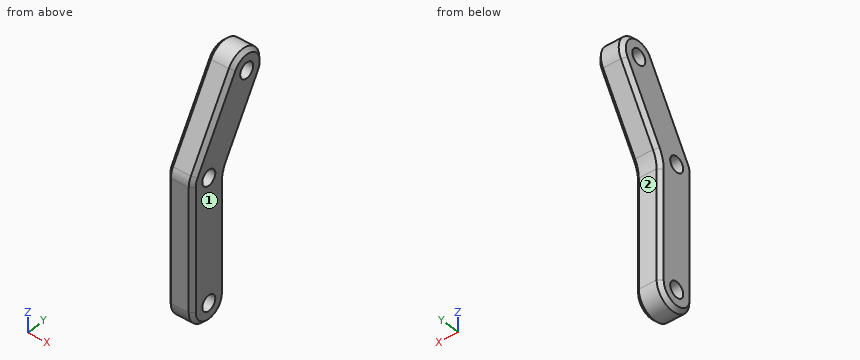
```python
from build123d import *

# Parameters (mm, degrees)
SKETCH_1_R      = 1.2
EXTRUDE_1_DEPTH = 2
FILLET_1_R      = 5
CHAMFER_1_SIZE  = 0.6


with BuildPart() as part:
    # Sketch 1 → Extrude 1 (new body, symmetric)
    with BuildSketch(Plane(origin=(0, 0, 0), x_dir=(0, 0, -1), z_dir=(1, 0, 0))):
        with BuildLine():
            Line((19, -3), (0, -3))
            ThreePointArc((0, -3), (-0.776457135, -2.897777479), (-1.5, -2.598076211))
            Line((-1.5, -2.598076211), (-13.624355653, 4.401923789))
            ThreePointArc((-13.624355653, 4.401923789), (-14.722431864, 8.5), (-10.624355653, 9.598076211))
            Line((-10.624355653, 9.598076211), (0.803847577, 3))
            Line((0.803847577, 3), (19, 3))
            ThreePointArc((19, 3), (22, 0), (19, -3))
        make_face()
        Circle(SKETCH_1_R, mode=Mode.SUBTRACT)
        with Locations((19, 0)):
            Circle(SKETCH_1_R, mode=Mode.SUBTRACT)
        with Locations((-12.124355653, 7)):
            Circle(SKETCH_1_R, mode=Mode.SUBTRACT)
    extrude(amount=EXTRUDE_1_DEPTH, both=True)

    # Fillet 1
    fillet_1_edges = [part.edges().sort_by_distance(p)[0] for p in [
        (0, 3, -0.803847577),
    ]]
    fillet(fillet_1_edges, radius=FILLET_1_R)

    # Chamfer 1
    chamfer_1_edges = [part.edges().sort_by_distance(p)[0] for p in [
        (-2, -2.897777479, 0.776457135),
        (2, 8.5, 14.722431864),
        (2, 6.633974596, 5.490381057),
        (2, 0, -22),
        (2, -3, -9.5),
        (-2, 3, -10.57179677),
        (2, 3, -10.57179677),
        (-2, 3.170370869, -0.849498314),
        (2, 3.170370869, -0.849498314),
        (2, -2.897777479, 0.776457135),
        (-2, -3, -9.5),
        (-2, 0, -22),
        (-2, 6.633974596, 5.490381057),
        (2, 0.901923789, 7.562177826),
        (-2, 8.5, 14.722431864),
        (-2, 0.901923789, 7.562177826),
    ]]
    chamfer(chamfer_1_edges, length=CHAMFER_1_SIZE)


solid = part.part
```
Work out the finished part from the listing and answer in its coordinate system (mm). Face numbers are marked on the shaded views. A direction names the side the tool comes from. Coordinates: 2 decimals unless noted, no trailing zeros. Order: outer loops, then holes, each group sorted by start corner. A loop starts at its lowest first (then second) coordinate and runs counter-clockwise, first axis right, second up. Notation, with made-up numbers: M 69,70 L 94,70 A29 ccw 94,104 Z; hole C 27.25,-4.75 d10. An arc over 180 degrees is marked long. Use CSV: the item, a comma, the result in double quotes.
1) Consider line 1 (Y direction, x = 1, z = -19); line 2 (Z direction, x = 0.3, y = 9.75); line 3 (Y direction, x = -1.15, z = -17). Determine where each line is inside the solid, lowest interval first. Write a range as [from, to].
Worked out:
line 1,"y = [-3, -1.2], [1.2, 3]"
line 2,"z = [10.93, 13.32]"
line 3,"y = [-3, 3]"
2) Section A-A on x = 1.05 is taken. Write down the section's boundary in (y, z).
Worked out:
outline,"M -3,-19 A3 ccw 3,-19 L 3,-2.14 A5 cw 3.67,0.36 L 9.6,10.62 A3 ccw 4.4,13.62 L -2.6,1.5 A3 ccw -3,0 Z; hole C 0,-19 d2.4; hole C 0,0 d2.4; hole C 7,12.12 d2.4"
3) Section C-C on y = 7 is taken. Write down the section's boundary in (x, z), plus the area to 3 significant figures.
Worked out:
outline,"M -2,7.32 L -1.4,6.12 L 1.4,6.12 L 2,7.32 L 2,10.92 L -2,10.92 Z; M -2,13.32 L 2,13.32 L 2,14.52 L 1.4,15.12 L -1.4,15.12 L -2,14.52 Z"
area,"25.3 mm^2"
4) For the marked faces 1 and 2, determine the directions among +Z, -Z, +X, -X, +Y, -Y from which every point of the face is accessible in a straight line to the end or side of a thin tool.
Worked out:
face 1,"+Z, -Z, +X, +Y, -Y"
face 2,"-Z, +X, -X, +Y"
5) Section D-D on z = 6 is taken. Write down the section's boundary in (x, y).
Worked out:
outline,"M -2,0.69 L -1.4,0 L 1.4,0 L 2,0.69 L 2,6.24 L 1.4,6.93 L -1.4,6.93 L -2,6.24 Z"
6) Section B-B on z = -10.5 is taken. Write down the section's boundary in (x, y).
Worked out:
outline,"M -2,-2.4 L -1.4,-3 L 1.4,-3 L 2,-2.4 L 2,2.4 L 1.4,3 L -1.4,3 L -2,2.4 Z"
7) Flat-ended cylindrical pins translate along their axes: pin 1 Ø2 at (x, z) = (0.5, -12) entering from +Y; pin 2 Ø2 at (y, z) = (0, -19) entering from +X. Find the tip coordinate at first contact, or state that the pin passes through.
Worked out:
pin 1,"stops at y = 3"
pin 2,"passes through"
